For this review, take the finished solid that the model builds, in its own axes (mm). A direction names the side the tool comes from. Give positions to 0.01 mm unless a question says otherwise; leave off trailing zeros. Order: outer loops, then holes, each group sorted by start corner. A loop starts at its lowest first (then second) coordinate and runs counter-clockwise, first axis right, second up. Notation, with made-up numbers: (88, 54.25) - (93, 54.25) arc R10 ccw to (93, 60.25) - close; hole circle Ø10 at (-6.5, 34.25). An arc over 180 degrees is marked (long way). Use a Markdown table: item, result. Add a question column.
1) Wall thickness on L1, parallel to X at y = 5.5, z = 16; L2, parallel to Z at x = 1, y = 1; L3, parallel to X at y = 4.25, z = 6.5: over which ranges is each line inside the solid? List them lowest first.
2) Machinability: for faces 4 (the face through (-45.22, 4.38, 44.7)), 5 (the face through (0, 7, 66.784)), 6 (the face through (49, 3.4, -44)), which of the approach directions +Z, -Z, +X, -X, +Y, -Y give a long, thin tool a straight path to every point of the face, cutting with its end or side? Answer none if there is none.
3) Mouldability with a two-part tool opening along X and no side actions: class faces 1 (the face through (45.543, 5.704, -46.075)), 2 (the face through (-48.07, 4.36, 48.64)), 3 (the face through (47.832, 8.439, 48.393)) as released by +X, released by -X, zero draft, split by the parting line, or undercut.
4) We need section A-A on x = -19. Write out the cut boundary in (y, z), then the cut area to 3 significant figures.
Autodesk Inventor part; units mm, degrees
ref_plane "작업 평면3" through (0, 4.4, 0) normal (0, -1, 0) x (1, 0, 0)
ref_plane "YZ Plane" through (0, 0, 0) normal (1, 0, 0) x (0, 1, 0)
ref_plane "XZ Plane" through (0, 0, 0) normal (0, 1, 0) x (-1, 0, 0)
sketch "스케치1" plane through (0, 0, 0) normal (0, 1, 0) x (-1, 0, 0)
  line L0 (-65.1838, 27) -> (-27, 65.1838)
  line L1 (-27, 65.1838) -> (27, 65.1838)
  line L2 (27, 65.1838) -> (65.1838, 27)
  line L3 (65.1838, 27) -> (65.1838, -27)
  line L4 (65.1838, -27) -> (27, -65.1838)
  line L5 (27, -65.1838) -> (-27, -65.1838)
  line L6 (-27, -65.1838) -> (-65.1838, -27)
  line L7 (-65.1838, -27) -> (-65.1838, 27)
  line L8 (68.3838, 28.3255) -> (68.3838, -28.3255)
  line L9 (68.3838, -28.3255) -> (28.3255, -68.3838)
  line L10 (28.3255, -68.3838) -> (-28.3255, -68.3838)
  line L11 (-28.3255, -68.3838) -> (-68.3838, -28.3255)
  line L12 (-68.3838, -28.3255) -> (-68.3838, 28.3255)
  line L13 (-68.3838, 28.3255) -> (-28.3255, 68.3838)
  line L14 (-28.3255, 68.3838) -> (28.3255, 68.3838)
  line L15 (28.3255, 68.3838) -> (68.3838, 28.3255)
  point P0 (0, 0)
  point P1 (0, 0)
  point P2 (0, 0)
  dimension "d0" = 54
  dimension "d1" = 3.2
extrude "돌출1" add sketch "스케치1" along normal blind 8.8 contours L0 L1 L2 L3 L4 L5 L6 L7 | L8 L9 L10 L11 L12 L13 L14 L15
sketch "스케치3" plane through (0, 0, 0) normal (0, -1, 0) x (1, 0, 0)
  line L0 (-26.8343, 64.7838) -> (26.8343, 64.7838)
  line L1 (26.8343, 64.7838) -> (64.7838, 26.8343)
  line L2 (64.7838, 26.8343) -> (64.7838, -26.8343)
  line L3 (64.7838, -26.8343) -> (26.8343, -64.7838)
  line L4 (26.8343, -64.7838) -> (-26.8343, -64.7838)
  line L5 (-26.8343, -64.7838) -> (-64.7838, -26.8343)
  line L6 (-64.7838, -26.8343) -> (-64.7838, 26.8343)
  line L7 (-64.7838, 26.8343) -> (-26.8343, 64.7838)
  line L8 (-27.6627, 66.7838) -> (27.6627, 66.7838)
  line L9 (27.6627, 66.7838) -> (66.7838, 27.6627)
  line L10 (66.7838, 27.6627) -> (66.7838, -27.6627)
  line L11 (66.7838, -27.6627) -> (27.6627, -66.7838)
  line L12 (27.6627, -66.7838) -> (-27.6627, -66.7838)
  line L13 (-27.6627, -66.7838) -> (-66.7838, -27.6627)
  line L14 (-66.7838, -27.6627) -> (-66.7838, 27.6627)
  line L15 (-66.7838, 27.6627) -> (-27.6627, 66.7838)
  line L16 (-28.3255, 68.3838) -> (28.3255, 68.3838)
  point P0 (0, 0)
  point P1 (0, 0)
  point P2 (0, 0)
  point P3 (0, 0)
  dimension "d9" = 2
  dimension "d144" = 1.6
extrude "돌출3" cut sketch "스케치3" against normal blind 3.4
sketch "스케치14" plane through (0, 0, 0) normal (0, -1, 0) x (1, 0, 0)
  line L0 (64.7838, 26.8343) -> (26.8343, 64.7838)
  line L1 (26.8343, 64.7838) -> (-26.8343, 64.7838)
  line L2 (-26.8343, 64.7838) -> (-64.7838, 26.8343)
  line L3 (-64.7838, 26.8343) -> (-64.7838, -26.8343)
  line L4 (-64.7838, -26.8343) -> (-26.8343, -64.7838)
  line L5 (-26.8343, -64.7838) -> (26.8343, -64.7838)
  line L6 (26.8343, -64.7838) -> (64.7838, -26.8343)
  line L7 (64.7838, -26.8343) -> (64.7838, 26.8343)
  point P0 (0, 0)
extrude "돌출16" cut sketch "스케치14" against normal blind 2.8
sketch "스케치15" plane through (0, 2.8, 0) normal (0, -1, 0) x (1, 0, 0)
  line L0 (-26.3373, 63.5838) -> (26.3373, 63.5838)
  line L1 (26.3373, 63.5838) -> (63.5838, 26.3373)
  line L2 (63.5838, 26.3373) -> (63.5838, -26.3373)
  line L3 (63.5838, -26.3373) -> (26.3373, -63.5838)
  line L4 (26.3373, -63.5838) -> (-26.3373, -63.5838)
  line L5 (-26.3373, -63.5838) -> (-63.5838, -26.3373)
  line L6 (-63.5838, -26.3373) -> (-63.5838, 26.3373)
  line L7 (-63.5838, 26.3373) -> (-26.3373, 63.5838)
  line L8 (-26.8343, 64.7838) -> (26.8343, 64.7838)
  point P0 (0, 0)
  point P1 (0, 0)
  dimension "d140" = 1.2
extrude "돌출17" cut sketch "스케치15" against normal up to surface (6 mm away)
ref_plane "작업 평면3" through (0, 4.4, 0) normal (0, -1, 0) x (1, 0, 0)
mirror "미러6" about plane through (0, 4.4, 0) normal (0, -1, 0) of "돌출3", "돌출16"
fillet "모깎기2" radius 1.2 16 edges at (0, 0, 68.3838) (-48.3546, 0, 48.3546) (-68.3838, 0, 0) (-48.3546, 0, -48.3546) (0, 0, -68.3838) (48.3546, 0, -48.3546) (68.3838, 0, 0) (48.3546, 0, 48.3546) (-48.3546, 8.8, 48.3546) (-68.3838, 8.8, 0) (-48.3546, 8.8, -48.3546) (0, 8.8, -68.3838) (48.3546, 8.8, -48.3546) (68.3838, 8.8, 0) (48.3546, 8.8, 48.3546) (0, 8.8, 68.3838)
properties part number "OV-PAM_ring_2"
Checked values:
| question | item | result |
|---|---|---|
| 1 | L1 | -68.38 to -66.78, -64.78 to -63.58, 63.58 to 64.78, 66.78 to 68.38 |
| 1 | L2 | -68.37 to -66.78, 66.78 to 68.37 |
| 1 | L3 | -68.38 to -63.58, 63.58 to 68.38 |
| 2 | face 4 | +Y, -Y |
| 2 | face 5 | +Y |
| 2 | face 6 | -Y |
| 3 | face 1 | undercut |
| 3 | face 2 | released by -X |
| 3 | face 3 | released by +X |
| 4 | outline | (0, -67.18) arc R1.2 ccw to (1.2, -68.38) - (7.6, -68.38) arc R1.2 ccw to (8.8, -67.18) - (8.8, -66.78) - (5.4, -66.78) - (5.4, -64.78) - (6, -64.78) - (6, -63.58) - (2.8, -63.58) - (2.8, -64.78) - (3.4, -64.78) - (3.4, -66.78) - (0, -66.78) - close; (0, 66.78) - (3.4, 66.78) - (3.4, 64.78) - (2.8, 64.78) - (2.8, 63.58) - (6, 63.58) - (6, 64.78) - (5.4, 64.78) - (5.4, 66.78) - (8.8, 66.78) - (8.8, 67.18) arc R1.2 ccw to (7.6, 68.38) - (1.2, 68.38) arc R1.2 ccw to (0, 67.18) - close |
| 4 | area | 42.6 mm² |
